Work out the finished part from the listing and answer in its coordinate system (mm). Face numbers are marked on the shaded views. A direction names the side the tool comes from. Give positions to 0.01 mm unless a question says otherwise; leave off trailing zeros. One line per question, with ' | ' between items. Start each with the question number.
1. Which of the six approach directions +Z, -Z, +X, -X, +Y, -Y give full straight-line access (tool end or side, diameter ignored) to the marked faces 1, 2 and 3?
2. Find the intervals of material crossed by line 1 (Z direction, x = 30, y = -51); line 2 (Z direction, x = 58, y = -19); line 3 (Y direction, x = 34.5, z = -10), in increasing order.
3. Each of these flat-tipped pins is pushed along its axis until it touches: pin 1 (9 mm diameter, centred on y = 99.14, z = -36.08, fed in from -X); pin 2 (3 mm diameter, centred on y = -85.5, z = 19.5, fed in from +X); pin 3 (2 mm diameter, centred on x = 59, y = -15, fed in from +Z); pin 4 (7 mm diameter, centred on y = -35.69, z = -80.16, fed in from -X). Where does it stop, or does it pass through?
4. For a pull along Y with two mould halves and no side action, classify the marked faces 4, 5 and 6 as released by +Y, released by -Y, zero draft, split by the parting line, or undercut.
5. Section A-A (x = 19.5) is taken. Give the number of separate pieces and of enclosed holes in the cut face, plus the area to 3 significant figures.
from build123d import *

# Parameters (mm, degrees)
F_8_0MM_DOWEL_HOLE1_D = 8
CIRPATTERN1_COUNT     = 18
SKETCH4_R             = 5
CUT_EXTRUDE1_DEPTH    = 179.080038185
SKETCH5_R             = 2.65
CUT_EXTRUDE2_DEPTH    = 169.337458695
CIRPATTERN2_COUNT     = 15
CHAMFER1_SIZE         = 2


with BuildPart() as part:
    # Sketch1 → Revolve1 (revolve)
    with BuildSketch(Plane.XY, mode=Mode.PRIVATE) as revolve1_sk:
        Polygon((0, 112.5), (80, 112.5), (80, 95), (55, 95), (55, 78.5), (43, 78.5), (43, 98.5), (0, 98.5), align=None)
    revolve(revolve1_sk.sketch.rotate(Axis((0, 0, 0), (1, 0, 0)), 90), axis=Axis((0, 0, 0), (1, 0, 0)))

    # 8.0mm Dowel Hole1 (through all)
    with Locations(Plane(origin=(0, 105.5, 0), x_dir=(0, 0, -1), z_dir=(-1, 0, 0))):
        with Locations((0, 0)):
            f_8_0mm_dowel_hole1 = Hole(F_8_0MM_DOWEL_HOLE1_D / 2)

    # CirPattern1: 8.0mm Dowel Hole1 ×18 about axis
    cirpattern1_axis = Axis((0, 0, 0), (1, 0, 0))
    for i in range(1, CIRPATTERN1_COUNT):
        add(f_8_0mm_dowel_hole1.rotate(cirpattern1_axis, i * 360 / CIRPATTERN1_COUNT), mode=Mode.SUBTRACT)

    # Sketch4 → Cut-Extrude1 (cut, through all)
    with BuildSketch(Plane.ZY):
        with Locations((105.5, 0)):
            Circle(SKETCH4_R)
        with Locations(Location((-105.5, 0, 0), (0, 0, 180))):
            Circle(SKETCH4_R)
    extrude(amount=-CUT_EXTRUDE1_DEPTH, mode=Mode.SUBTRACT)

    # Sketch5 → Cut-Extrude2 (cut, through all)
    with BuildSketch(Plane(origin=(55, 0, 0), x_dir=(0, 0, -1), z_dir=(1, 0, 0))):
        with Locations((87.75, 0)):
            Circle(SKETCH5_R)
    cut_extrude2 = extrude(amount=-CUT_EXTRUDE2_DEPTH, mode=Mode.SUBTRACT)

    # CirPattern2: Cut-Extrude2 ×15 about axis
    cirpattern2_axis = Axis((0, 0, 0), (1, 0, 0))
    for i in range(1, CIRPATTERN2_COUNT):
        add(cut_extrude2.rotate(cirpattern2_axis, i * 360 / CIRPATTERN2_COUNT), mode=Mode.SUBTRACT)

    # Chamfer1
    chamfer1_edges = [part.edges().sort_by_distance(p)[0] for p in [
        (43, 0, -78.5),
        (55, 0, -78.5),
    ]]
    chamfer(chamfer1_edges, length=CHAMFER1_SIZE)


solid = part.part
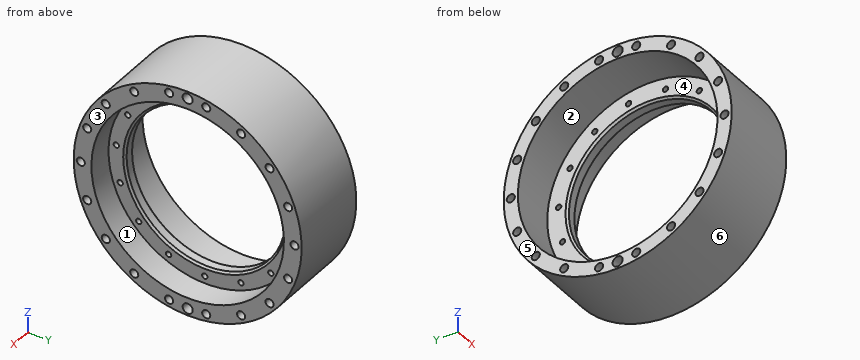
Conclusion:
1) face 1: +X | face 2: -X | face 3: +Z, -Z, +X, +Y, -Y
2) line 1: -100.28 to -94.96, -87.77 to -84.27, 84.27 to 87.77, 94.96 to 100.28 | line 2: -110.88 to -107.84, -99.96 to -93.08, 93.08 to 99.96, 107.84 to 110.88 | line 3: -112.05 to -97.99, 97.99 to 112.05
3) pin 1: x = 0 | pin 2: x = 55 | pin 3: z = 111.63 | pin 4: x = 43
4) face 4: undercut | face 5: zero draft | face 6: split by the parting line
5) separate pieces: 1 | enclosed holes: 21 | area: 8,220 mm²
